The model under review builds one solid part; all positions refer to its coordinate system, in mm. A direction names the side the tool comes from. Round coordinates to 2 decimals unless told otherwise and drop trailing zeros. Loops run counter-clockwise (first coordinate to the right, second up) from the corner with the lowest first, then second, coordinate; pieces in that order, holes last. Notation, with made-up numbers: M 53,-5 L 108,-5 A22 cw 108,5 Z; hole C -32.75,5.25 d3. An arc over 180 degrees is marked long. Answer as a JSON object with one key per item and string values. Group by question number.
Item 1: Consider section B-B (y = 33.5). Give the boundary of the cut face in (x, z).
Item 2: Tool access review of faces 1 (the face through (-1, 1, 0)), 2 (the face through (-1, -50.8, 62)), 3 (the face through (0, 1, 5.08)), 4 (the face through (-38.1, -1, 62)), 5 (the face through (38.1, -1, 62)): name each direction out of +Z, -Z, +X, -X, +Y, -Y from which nothing blocks a thin tool from reaching the whole face with its end or side.
Item 3: The part is to be moulded in two halves that separate along Y. For faces 6 (the face through (-41, 0, 55.88)), 7 (the face through (0, -46.99, 36)), 8 (the face through (-1, 50.8, 62)), say which applies: +Y half, -Y half, draft (parallel to the pull), parting line (faces both ways), or undercut.
Item 4: To check wall thickness, follow line 1 (X direction, y = 32, z = 65.5); line 2 (Y direction, x = 25, z = 14.5); line 3 (X direction, y = 40.5, z = 47). State the ranges of each line that lie inside material, in increasing order.
Item 5: Consider section D-D (z = 61). Give the boundary of the cut face in (x, y), and give its area (3 significant figures).
Item 6: Consider section A-A (z = 10). Give the boundary of the cut face in (x, y), and give its area (3 significant figures).
Item 7: Consider section C-C (x = -29). Give the boundary of the cut face in (y, z).
Item 8: Insertion check: P1, Ø3, axis at x = 8.5, z = 58, coming from the +Y side; P2, Ø6.5, axis at y = 23.5, z = 63, coming from the +X side; P3, Ø10, axis at x = -11.5, z = 62.5, coming from the -Y side; P4, Ø10, axis at y = 0, z = 59.5, coming from the -X side. Each pin has a flat end and moves straight along its axis. Give the tip position at first contact, or say it passes through.
```python
from build123d import *

# Parameters (mm, degrees)
F0_W     = 76.2
F0_H     = 101.6
F0_W_2   = 68.58
F0_H_2   = 93.98
F1_DEPTH = 68.58
F0_W_3   = 83.82
F0_H_3   = 109.22
F2_DEPTH = 55.88
F3_W     = 68.58
F3_H     = 93.98
F4_DEPTH = 5.08


with BuildPart() as f1:
    # F0 (on Top) → F1 (new body)
    with BuildSketch(Plane.XY):
        Rectangle(F0_W, F0_H)
        Rectangle(F0_W_2, F0_H_2, mode=Mode.SUBTRACT)
    extrude(amount=F1_DEPTH)

    # F0 (on Top) → F2 (join)
    with BuildSketch(Plane.XY):
        Rectangle(F0_W_3, F0_H_3)
        Rectangle(F0_W, F0_H, mode=Mode.SUBTRACT)
    extrude(amount=F2_DEPTH)

    # F3 (on Top) → F4 (join)
    with BuildSketch(Plane.XY):
        Rectangle(F3_W, F3_H)
    extrude(amount=F4_DEPTH)


solid = f1.part
```
Geometry results:
{
 "1": {"outline": "M -41.91,0 L 41.91,0 L 41.91,55.88 L 38.1,55.88 L 38.1,68.58 L 34.29,68.58 L 34.29,5.08 L -34.29,5.08 L -34.29,68.58 L -38.1,68.58 L -38.1,55.88 L -41.91,55.88 Z"},
 "2": {"face 1": "-Z, +X, -X, +Y, -Y", "face 2": "+Z, +X, -X, -Y", "face 3": "+Z", "face 4": "+Z, -X, +Y, -Y", "face 5": "+Z, +X, +Y, -Y"},
 "3": {"face 6": "draft", "face 7": "undercut", "face 8": "+Y half"},
 "4": {"line 1": "x = -38.1 to -34.29, 34.29 to 38.1", "line 2": "y = -54.61 to -46.99, 46.99 to 54.61", "line 3": "x = -41.91 to -34.29, 34.29 to 41.91"},
 "5": {"outline": "M -38.1,-50.8 L 38.1,-50.8 L 38.1,50.8 L -38.1,50.8 Z; hole M -34.29,-46.99 L 34.29,-46.99 L 34.29,46.99 L -34.29,46.99 Z", "area": "1,300 mm^2"},
 "6": {"outline": "M -41.91,-54.61 L 41.91,-54.61 L 41.91,54.61 L -41.91,54.61 Z; hole M -34.29,-46.99 L 34.29,-46.99 L 34.29,46.99 L -34.29,46.99 Z", "area": "2,710 mm^2"},
 "7": {"outline": "M -54.61,0 L 54.61,0 L 54.61,55.88 L 50.8,55.88 L 50.8,68.58 L 46.99,68.58 L 46.99,5.08 L -46.99,5.08 L -46.99,68.58 L -50.8,68.58 L -50.8,55.88 L -54.61,55.88 Z"},
 "8": {"P1": "stops at y = 50.8", "P2": "stops at x = 38.1", "P3": "stops at y = -50.8", "P4": "stops at x = -41.91"}
}
